Input: dimensioned drawing with shaded views. Units: mm. Origin: part minimum x, y, z. A direction names the side the tool comes from. Give positions to 0.01 mm unless a question says otherwise; leave off trailing zeros. Loops run counter-clockwise (first coordinate to the right, second up) from the corner with the lowest first, then second, coordinate; pieces in that order, holes last.
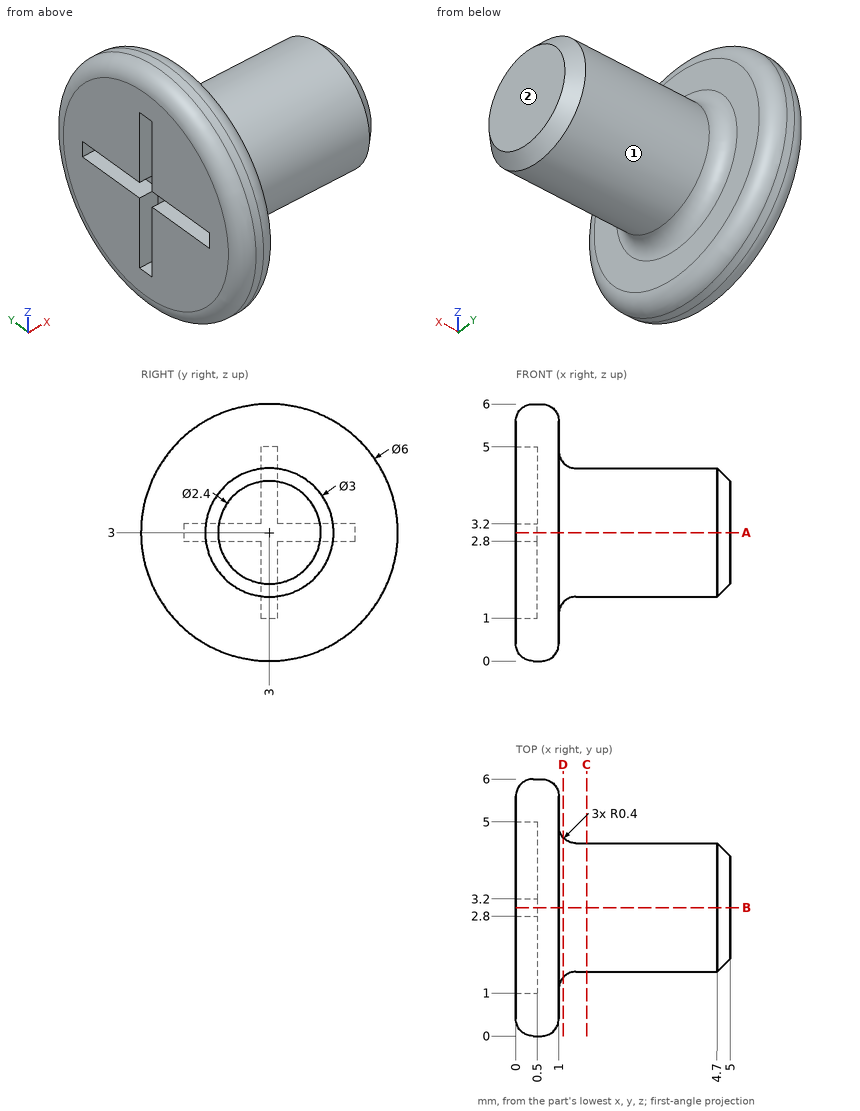
(1) First-contact query: pin 1 (1.5 mm diameter, centred on x = 4.5, z = 2.5, fed in from -Y); pin 2 (0.6 mm diameter, centred on x = 0, z = 4.5, fed in from -Y); pin 3 (0.6 mm diameter, centred on x = 0, z = 4, fed in from +Y). Flat tips, straight axial feed; report the tip coordinate or a pass-through.
A:
pin 1: stops at y = 1.5
pin 2: stops at y = 0.34
pin 3: stops at y = 5.85
(2) Reachability of the marked faces 1 and 2 from +Z, -Z, +X, -X, +Y, -Y: full face, straight path, thin tool, end or side. Return the list, or none.
A:
face 1: +X
face 2: +Z, -Z, +X, +Y, -Y
(3) Ray query, line 1 along X through (y, z) = (0.8, 3.05); line 2 along X through (y, z) = (3.05, 2.4); line 3 along Z through (x, y) = (3.65, 3.75). Return the intervals inside material, ascending.
A:
line 1: x = 0 to 1
line 2: x = 0.5 to 5
line 3: z = 1.7 to 4.3
(4) Section A-A, the plane z = 3. Return the cut outline in (x, y), then the cut area to 3 significant figures.
A:
outline: (0, 0.4) arc R0.4 ccw to (0.4, 0) - (0.6, 0) arc R0.4 ccw to (1, 0.4) - (1, 1.1) arc R0.4 cw to (1.4, 1.5) - (4.7, 1.5) - (5, 1.8) - (5, 4.2) - (4.7, 4.5) - (1.4, 4.5) arc R0.4 cw to (1, 4.9) - (1, 5.6) arc R0.4 ccw to (0.6, 6) - (0.4, 6) arc R0.4 ccw to (0, 5.6) - (0, 5) - (0.5, 5) - (0.5, 1) - (0, 1) - close
area: 15.8 mm2
(5) Section C-C, the plane x = 1.65. Return the cut outline in (y, z).
A:
outline: circle Ø3 at (3, 3)
(6) Section D-D, the plane x = 1.1. Return the cut outline in (y, z).
A:
outline: circle Ø3.27 at (3, 3)
